```python
from build123d import *

# Parameters (mm, degrees)
SKETCH1_R                = 20
BOSS_EXTRUDE1_DEPTH      = 10
CUT_EXTRUDE1_DEPTH       = 2.5
BOSS_EXTRUDE2_DEPTH      = 10
BOSS_EXTRUDE3_START      = 6
SKETCH6_R                = 12.5
BOSS_EXTRUDE3_DEPTH      = 6
BOSS_EXTRUDE4_DEPTH      = 10
BOSS_EXTRUDE4_DEPTH_BACK = 20
SKETCH8_R                = 2.5
CUT_EXTRUDE2_DEPTH       = 99.517232015
SKETCH9_R                = 12.5
CUT_EXTRUDE3_DEPTH       = 2.5
SKETCH10_W               = 45
SKETCH10_H               = 15
BOSS_EXTRUDE5_DEPTH      = 9.95
SKETCH11_W               = 45
SKETCH11_H               = 15
BOSS_EXTRUDE6_DEPTH      = 9.95
SKETCH12_R               = 47.5
CUT_EXTRUDE5_DEPTH       = 9.95


with BuildPart() as part:
    # Sketch1 → Boss-Extrude1 (new body)
    with BuildSketch(Plane(origin=(0, 0, 0), x_dir=(1, 0, 0), z_dir=(0, 1, 0))):
        with Locations(Location((0, 0, 0), (0, 0, 270))):
            Circle(SKETCH1_R)
    extrude(amount=BOSS_EXTRUDE1_DEPTH)

    # Sketch2 → Cut-Extrude1 (cut)
    with BuildSketch(Plane(origin=(0, 10, 0), x_dir=(1, 0, 0), z_dir=(0, 1, 0))):
        with BuildLine():
            Line((-2.683281573, 3.1), (2.683281573, 3.1))
            ThreePointArc((2.683281573, 3.1), (0, -4.1), (-2.683281573, 3.1))
        make_face()
    extrude(amount=-CUT_EXTRUDE1_DEPTH, mode=Mode.SUBTRACT)

    # Sketch3 → Boss-Extrude2 (add)
    with BuildSketch(Plane(origin=(0, 0, 0), x_dir=(1, 0, 0), z_dir=(0, 1, 0))):
        with BuildLine():
            Line((-17.5, 59.682458366), (-17.5, 9.682458366))
            ThreePointArc((-17.5, 9.682458366), (0, 20), (17.5, 9.682458366))
            Line((17.5, 9.682458366), (17.5, 59.682458366))
            Line((17.5, 59.682458366), (-17.5, 59.682458366))
        make_face()
    extrude(amount=BOSS_EXTRUDE2_DEPTH)

    # Sketch6 → Boss-Extrude3 (add)
    with BuildSketch(Plane(origin=(0, 10, 0), x_dir=(1, 0, 0), z_dir=(0, 1, 0)).offset(BOSS_EXTRUDE3_START)):
        with Locations(Location((0, 0, 0), (0, 0, 270))):
            Circle(SKETCH6_R)
        with BuildLine():
            Line((-2.683281573, 3.1), (2.683281573, 3.1))
            ThreePointArc((2.683281573, 3.1), (0, -4.1), (-2.683281573, 3.1))
        make_face(mode=Mode.SUBTRACT)
    extrude(amount=-BOSS_EXTRUDE3_DEPTH)

    # Sketch7 → Boss-Extrude4 (add, two sides: drawn at the far end of the back side and taken through both)
    with BuildSketch(Plane(origin=(0, 0, -59.682458366), x_dir=(-1, 0, 0), z_dir=(0, 0, -1)).offset(-BOSS_EXTRUDE4_DEPTH_BACK)):
        Polygon((-32.5, 0), (-32.5, 25), (-22.5, 25), (-22.5, 10), (22.5, 10), (22.5, 25), (32.5, 25), (32.5, 0), align=None)
    extrude(amount=BOSS_EXTRUDE4_DEPTH + BOSS_EXTRUDE4_DEPTH_BACK)

    # Sketch8 → Cut-Extrude2 (cut, through all)
    with BuildSketch(Plane.ZY.offset(32.5)):
        with Locations((-54.682458366, 17.5)):
            Circle(SKETCH8_R)
    extrude(amount=-CUT_EXTRUDE2_DEPTH, mode=Mode.SUBTRACT)

    # Sketch9 → Cut-Extrude3 (cut)
    with BuildSketch(Plane(origin=(0, 16, 0), x_dir=(1, 0, 0), z_dir=(0, 1, 0))):
        with Locations(Location((0, 0, 0), (0, 0, 270))):
            Circle(SKETCH9_R)
    extrude(amount=-CUT_EXTRUDE3_DEPTH, mode=Mode.SUBTRACT)

    # Sketch10 → Boss-Extrude5 (add)
    with BuildSketch(Plane(origin=(0, 0, -69.682458366), x_dir=(-1, 0, 0), z_dir=(0, 0, -1))):
        with Locations((0, 17.5)):
            Rectangle(SKETCH10_W, SKETCH10_H)
    extrude(amount=-BOSS_EXTRUDE5_DEPTH)

    # Sketch11 → Boss-Extrude6 (add)
    with BuildSketch(Plane.XY.offset(-39.682458366)):
        with Locations((0, 17.5)):
            Rectangle(SKETCH11_W, SKETCH11_H)
    extrude(amount=-BOSS_EXTRUDE6_DEPTH)

    # Sketch12 → Cut-Extrude5 (cut)
    with BuildSketch(Plane(origin=(0, 0, -69.682458366), x_dir=(-1, 0, 0), z_dir=(0, 0, -1))):
        with Locations((0, 70)):
            Circle(SKETCH12_R)
    extrude(amount=-CUT_EXTRUDE5_DEPTH, mode=Mode.SUBTRACT)


solid = part.part
```
Build history of the part. All positions in model axes, mm. A direction names the side the tool comes from. Give positions to 0.01 mm unless a question says otherwise; leave off trailing zeros. Loops run counter-clockwise (first coordinate to the right, second up) from the corner with the lowest first, then second, coordinate; pieces in that order, holes last. Notation, with made-up numbers: (-27.75, 68) -> (5.25, 68) arc R17 ccw to (5.25, 91) -> close; hole circle Ø2 at (22, 34.5). An arc over 180 degrees is marked (long way). One line per question, with ' | ' between items.
Q1. Drop flat-ended pins along their axis: pin 1 (11 mm diameter, centred on x = -10, z = -54, fed in from +Y); pin 2 (2 mm diameter, centred on x = -5, z = -20.5, fed in from +Y); pin 3 (1.5 mm diameter, centred on x = -9.5, z = -59.5, fed in from +Y); pin 4 (6 mm diameter, centred on x = 0, y = 11.5, fed in from +Z). Give the stop position or say it passes through.
Filled sheet:
pin 1: stops at y = 25 | pin 2: stops at y = 10 | pin 3: stops at y = 23.61 | pin 4: stops at z = 20
Q2. Pull direction X, two halves, no side cores. Call faces 1 (the cylindrical face through (0.1, 10.5, 4.1)), 2 (the flat face through (0, 10, -16)), 3 (the flat face through (22.5, 16, -52)), 4 (the flat face through (-17.5, 5, -25)): pulls with the +X half, pulls with the -X half, needs draft (parallel to the pull), parting line crosses it, or undercut.
Filled sheet:
face 1: undercut | face 2: needs draft | face 3: undercut | face 4: pulls with the -X half
Q3. Drill centre lines: line 1 along X through (y, z) = (9.85, 0); line 2 along X through (y, z) = (10.6, 0); line 3 along Z through (x, y) = (-20, 12.5). Where is each one in solid material? Low to high. Write a range as [from, to].
Filled sheet:
line 1: x = [-20, -4.1], [4.1, 20] | line 2: x = [-12.5, -4.1], [4.1, 12.5] | line 3: z = [-69.68, -59.73], [-49.63, -39.68]
Q4. Cut at A-A, the plane y = 17.5. Write the cut outline in (x, z), plus the area to 3 significant figures.
Filled sheet:
outline: (-32.5, -69.68) -> (32.5, -69.68) -> (32.5, -57.18) -> (22.5, -57.18) -> (22.5, -59.73) -> (-22.5, -59.73) -> (-22.5, -57.18) -> (-32.5, -57.18) -> close; (-32.5, -52.18) -> (-22.5, -52.18) -> (-22.5, -49.63) -> (22.5, -49.63) -> (22.5, -52.18) -> (32.5, -52.18) -> (32.5, -39.68) -> (-32.5, -39.68) -> close | area: 1,400 mm²
Q5. Cut at B-B, the plane x = -27. Write the cut outline in (y, z).
Filled sheet:
outline: (0, -69.68) -> (25, -69.68) -> (25, -39.68) -> (0, -39.68) -> close; hole circle Ø5 at (17.5, -54.68)
Q6. Cut at D-D, the plane y = 3.25. Write the cut outline in (x, z), plus the area to 3 significant figures.
Filled sheet:
outline: (-32.5, -69.68) -> (32.5, -69.68) -> (32.5, -39.68) -> (17.5, -39.68) -> (17.5, -9.68) arc R20 ccw (long way) to (-17.5, -9.68) -> (-17.5, -39.68) -> (-32.5, -39.68) -> close | area: 4,000 mm²
Q7. Tool access for faces 5 (the flat face through (17.5, 5, -24)), 6 (the cylindrical face through (3.755, 11.774, 11.923)), 7 (the flat face through (-5, 13.5, 0)): list every direction of +Z, -Z, +X, -X, +Y, -Y with a clear straight run to the whole face (end or side of a thin tool).
Filled sheet:
face 5: +X, +Y, -Y | face 6: +Y | face 7: +Z, +X, -X, +Y
Q8. Cut at C-C, the plane z = 0. Write the cut outline in (x, y), plus the area to 3 significant figures.
Filled sheet:
outline: (-20, 0) -> (20, 0) -> (20, 10) -> (12.5, 10) -> (12.5, 13.5) -> (4.1, 13.5) -> (4.1, 7.5) -> (-4.1, 7.5) -> (-4.1, 13.5) -> (-12.5, 13.5) -> (-12.5, 10) -> (-20, 10) -> close | area: 438 mm²
